Read the model definition and answer for the solid it produces. Units are mm, in the model's axes. A direction names the side the tool comes from. Coordinates: 2 decimals unless noted, no trailing zeros. Use a Markdown table: item, result.
from build123d import *

# Parameters (mm, degrees)
BOSS_EXTRUDE1_DEPTH         = 1060
CUT_EXTRUDE1_DEPTH          = 800
SKETCH5_W                   = 10.426623187
SKETCH5_H                   = 125.292137731
BOSS_EXTRUDE2_DEPTH         = 950
SKETCH6_W                   = 7.435137382
SKETCH6_H                   = 64.029540506
BOSS_EXTRUDE3_DEPTH         = 50
LPATTERN1_COUNT             = 10
LPATTERN1_PITCH             = 100
CUT_EXTRUDE3_DEPTH          = 10
CUT_EXTRUDE3_DEPTH_BACK     = 100
CUT_EXTRUDE2_START          = -300
SKETCH3_W                   = 37.098457344
SKETCH3_H                   = 15
CUT_EXTRUDE2_DEPTH          = 1000
SKETCH7_W                   = 41.986295648
SKETCH7_H                   = 14.210937294
BOSS_EXTRUDE4_DEPTH         = 30
SKETCH8_R                   = 3.874254892
CUT_EXTRUDE4_DEPTH          = 30
SKETCH_1_R                  = 3.167509586
CUT_EXTRUDE_1_DEPTH         = 10
PATTERN_LINEAR_1_COUNT      = 2
PATTERN_LINEAR_1_PITCH      = 44
PATTERN_LINEAR_1_COUNT_DIR2 = 2
PATTERN_LINEAR_1_PITCH_DIR2 = 1000
SKETCH9_R                   = 6.088028913
CUT_EXTRUDE5_DEPTH          = 10
LPATTERN2_COUNT             = 2
LPATTERN2_PITCH             = 1005
CUT_EXTRUDE6_DEPTH          = 10


with BuildPart() as part:
    # Sketch1 → Boss-Extrude1 (new body)
    with BuildSketch(Plane.XY):
        with BuildLine():
            Line((-31.555119126, 31.290150882), (-37.853807036, 37.718722311))
            Line((-37.853807036, 37.718722311), (-39.853807036, 37.718722311))
            Line((-39.853807036, 37.718722311), (-46.282378465, 31.420034401))
            Line((-46.282378465, 31.420034401), (-46.282378465, 30.420034401))
            Line((-46.282378465, 30.420034401), (-51.282378465, 30.420034401))
            Line((-51.282378465, 30.420034401), (-51.282378465, 31.420034401))
            Line((-51.282378465, 31.420034401), (-96.206307824, 31.420034401))
            Line((-96.206307824, 31.420034401), (-101.105287309, 36.420034401))
            Line((-101.105287309, 36.420034401), (-103.105287309, 36.420034401))
            Line((-103.105287309, 36.420034401), (-108.055034777, 31.470286932))
            Line((-108.055034777, 31.470286932), (-108.055034777, 30.420034401))
            Line((-108.055034777, 30.420034401), (-113.055034777, 30.420034401))
            Line((-113.055034777, 30.420034401), (-113.055034777, 31.420034401))
            Line((-113.055034777, 31.420034401), (-131.555034777, 31.420034401))
            Line((-131.555034777, 31.420034401), (-131.555034777, 21.420034401))
            Line((-131.555034777, 21.420034401), (-87.349569261, 21.420034401))
            ThreePointArc((-87.349569261, 21.420034401), (-68.862935324, 14.835575372), (-58.701074529, -1.95273366))
            Line((-58.701074529, -1.95273366), (-58.701074529, -92.579965599))
            ThreePointArc((-58.701074529, -92.579965599), (-60.165540623, -96.115499505), (-63.701074529, -97.579965599))
            Line((-63.701074529, -97.579965599), (-108.009983562, -97.579965599))
            Line((-108.009983562, -97.579965599), (-108.009983562, -107.579965599))
            Line((-108.009983562, -107.579965599), (-31.195424592, -107.579965599))
            Line((-31.195424592, -107.579965599), (-31.195424592, -97.579965599))
            Line((-31.195424592, -97.579965599), (-43.701074529, -97.579965599))
            ThreePointArc((-43.701074529, -97.579965599), (-47.236608435, -96.115499505), (-48.701074529, -92.579965599))
            Line((-48.701074529, -92.579965599), (-48.701074529, 21.290150882))
            Line((-48.701074529, 21.290150882), (-31.555119126, 21.290150882))
            Line((-31.555119126, 21.290150882), (-31.555119126, 31.290150882))
        make_face()
    extrude(amount=BOSS_EXTRUDE1_DEPTH)

    # Sketch2 → Cut-Extrude1 (cut)
    with BuildSketch(Plane(origin=(0, 20.764722339, 0), x_dir=(1, 0, 0), z_dir=(0, 1, 0))):
        with BuildLine():
            Line((-84.170689991, 100), (-77.170689991, 100))
            ThreePointArc((-77.170689991, 100), (-70.099622179, 97.071067812), (-67.170689991, 90))
            Line((-67.170689991, 90), (-67.170689991, -890))
            ThreePointArc((-67.170689991, -890), (-70.099622179, -897.071067812), (-77.170689991, -900))
            Line((-77.170689991, -900), (-84.170689991, -900))
            ThreePointArc((-84.170689991, -900), (-91.241757803, -897.071067812), (-94.170689991, -890))
            Line((-94.170689991, -890), (-94.170689991, 90))
            ThreePointArc((-94.170689991, 90), (-91.241757803, 97.071067812), (-84.170689991, 100))
        make_face()
    extrude(amount=CUT_EXTRUDE1_DEPTH, mode=Mode.SUBTRACT)

    # Sketch5 → Boss-Extrude2 (add)
    with BuildSketch(Plane(origin=(0, 0, 0), x_dir=(-1, 0, 0), z_dir=(0, 0, -1))):
        with Locations((100.133130522, -34.849417223)):
            Rectangle(SKETCH5_W, SKETCH5_H)
    extrude(amount=-BOSS_EXTRUDE2_DEPTH)

    # Sketch6 → Boss-Extrude3 (add)
    with BuildSketch(Plane.ZY.offset(105.346442115)):
        with Locations((3.717568691, -15.430068515)):
            Rectangle(SKETCH6_W, SKETCH6_H)
    boss_extrude3 = extrude(amount=-BOSS_EXTRUDE3_DEPTH)

    # LPattern1: Boss-Extrude3 ×10
    with Locations(*[(0, 0, i * LPATTERN1_PITCH) for i in range(1, LPATTERN1_COUNT)]):
        add(boss_extrude3)

    # Sketch4 → Cut-Extrude3 (cut, two sides)
    with BuildSketch(Plane(origin=(-31.555119126, 0, 0), x_dir=(0, 0, -1), z_dir=(1, 0, 0))) as cut_extrude3_sk:
        with BuildLine():
            Line((-910, -97.579965599), (-910, -107.579965599))
            Line((-910, -107.579965599), (-910, -177.956634241))
            Line((-910, -177.956634241), (-70, -177.956634241))
            Line((-70, -177.956634241), (-70, -97.579965599))
            ThreePointArc((-70, -97.579965599), (-121.056751887, -63.823667059), (-180.068799532, -47.579965599))
            Line((-180.068799532, -47.579965599), (-800, -47.579965599))
            ThreePointArc((-800, -47.579965599), (-859.23910305, -63.253938888), (-910, -97.579965599))
        make_face()
    extrude(amount=CUT_EXTRUDE3_DEPTH, mode=Mode.SUBTRACT)
    extrude(cut_extrude3_sk.sketch, amount=-CUT_EXTRUDE3_DEPTH_BACK, mode=Mode.SUBTRACT)

    # Sketch3 → Cut-Extrude2 (cut)
    with BuildSketch(Plane.XY.offset(1060).offset(CUT_EXTRUDE2_START)):
        with Locations((-77.250303201, 13.920034401)):
            Rectangle(SKETCH3_W, SKETCH3_H)
    extrude(amount=-CUT_EXTRUDE2_DEPTH, mode=Mode.SUBTRACT)

    # Sketch7 → Boss-Extrude4 (add)
    with BuildSketch(Plane(origin=(0, 0, 0), x_dir=(-1, 0, 0), z_dir=(0, 0, -1))):
        with Locations((78.756733265, -0.685434246)):
            Rectangle(SKETCH7_W, SKETCH7_H)
    extrude(amount=-BOSS_EXTRUDE4_DEPTH)

    # Sketch8 → Cut-Extrude4 (cut)
    with BuildSketch(Plane(origin=(0, 6.420034401, 0), x_dir=(1, 0, 0), z_dir=(0, 1, 0))):
        with Locations((-79.789069173, -14.972288239)):
            Circle(SKETCH8_R)
    extrude(amount=-CUT_EXTRUDE4_DEPTH, mode=Mode.SUBTRACT)

    # Эскиз1 → Вырез-Вытянуть1 (cut)
    with BuildSketch(Plane(origin=(-48.701074529, 0, 0), x_dir=(0, 0, -1), z_dir=(1, 0, 0))):
        with Locations((-45, 3.290150882)):
            Circle(SKETCH_1_R)
    cut_extrude_1 = extrude(amount=-CUT_EXTRUDE_1_DEPTH, mode=Mode.SUBTRACT)

    # Линейный массив1: Cut-Extrude 1 2 × 2
    with Locations(*[(0, -i * PATTERN_LINEAR_1_PITCH, j * PATTERN_LINEAR_1_PITCH_DIR2) for i in range(PATTERN_LINEAR_1_COUNT) for j in range(PATTERN_LINEAR_1_COUNT_DIR2) if (i, j) != (0, 0)]):
        add(cut_extrude_1, mode=Mode.SUBTRACT)

    # Sketch9 → Cut-Extrude5 (cut)
    with BuildSketch(Plane.XZ.offset(107.579965599)):
        with Locations((-75.432174638, 36.066091654)):
            Circle(SKETCH9_R)
    cut_extrude5 = extrude(amount=-CUT_EXTRUDE5_DEPTH, mode=Mode.SUBTRACT)

    # LPattern2: Cut-Extrude5 ×2
    with Locations(*[(0, 0, i * LPATTERN2_PITCH) for i in range(1, LPATTERN2_COUNT)]):
        add(cut_extrude5, mode=Mode.SUBTRACT)

    # Sketch10 → Cut-Extrude6 (cut)
    with BuildSketch(Plane.XZ.offset(107.579965599)):
        with BuildLine():
            Line((-81.818611273, 1041.066091654), (-81.818611273, 1067.229436247))
            ThreePointArc((-81.818611273, 1067.229436247), (-75.432174638, 1073.615872882), (-69.045738002, 1067.229436247))
            Line((-69.045738002, 1067.229436247), (-69.045738002, 1041.066091654))
            ThreePointArc((-69.045738002, 1041.066091654), (-75.432174638, 1034.679655018), (-81.818611273, 1041.066091654))
        make_face()
    extrude(amount=-CUT_EXTRUDE6_DEPTH, mode=Mode.SUBTRACT)


solid = part.part
(1) For faces 4 (the flat face through (-40, 21.29, 523)), 5 (the cylindrical face through (-53.561, -62.899, 858.454)), 6 (the flat face through (-77, -21, 407.435)), determine the directions among +Z, -Z, +X, -X, +Y, -Y from which every point of the face is accessible in a straight line to the end or side of a thin tool.
Report:
| item | result |
|---|---|
| face 4 | +Z, -Z, +X |
| face 5 | +X, -X, -Y |
| face 6 | -Y |
(2) Each of these flat-tipped pins is pushed along its axis until it touches: P1, Ø0.5, axis at y = 31, z = 638.5, coming from the +X side; P2, Ø5, axis at x = -114.5, z = 889.5, coming from the +Y side; P3, Ø6, axis at x = -45, z = 805.5, coming from the -Y side; P4, Ø5, axis at y = -40.71, z = 1045, coming from the -X side. Where does it stop, or does it pass through?
Report:
| item | result |
|---|---|
| P1 | stops at x = -31.56 |
| P2 | stops at y = 31.42 |
| P3 | stops at y = 21.29 |
| P4 | passes through |
(3) Straight lines are drawn through the part: L1, parallel to Y at x = -52.25, z = 45; L2, parallel to Z at x = -83.5, y = 13.5; L3, parallel to X at y = -37, z = 410.5. For each, find the intervals that lie inside material, in ascending order.
Report:
| item | result |
|---|---|
| L1 | y = -107.58 to -43.88, -37.54 to 0.12, 6.46 to 31.42 |
| L2 | z = 800 to 807.44, 900 to 907.44 |
| L3 | x = -105.35 to -94.92, -58.7 to -48.7 |
(4) The mould has two halves that part along Y. Classify faces 1 (the flat face through (-86, -97.58, 35)), 2 (the flat face through (-122, 31.42, 523)), 3 (the flat face through (-77, -21, 400)): pulls with the +Y half, pulls with the -Y half, needs draft (parallel to the pull), parting line crosses it, or undercut.
Report:
| item | result |
|---|---|
| face 1 | undercut |
| face 2 | pulls with the +Y half |
| face 3 | needs draft |
